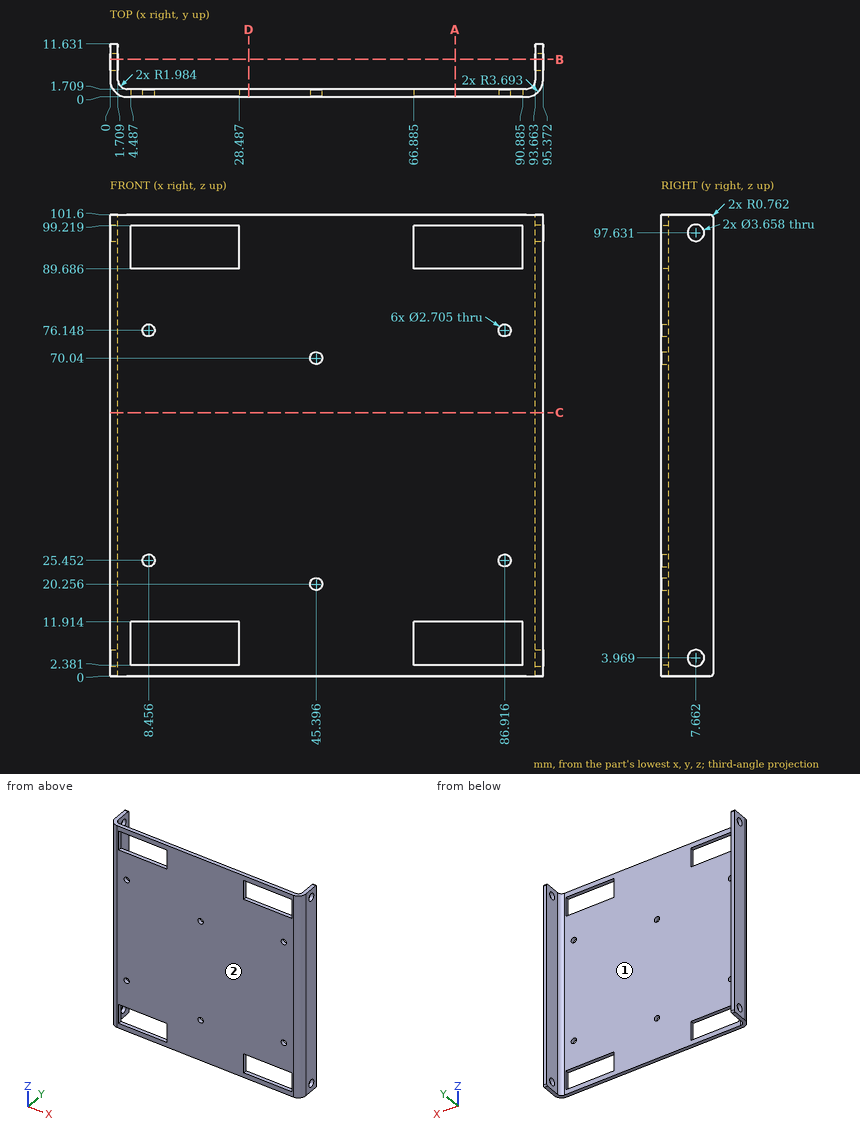
Verification items for this drawing (mm, ordinates from the low corner). Coordinates: 2 decimals unless noted, no trailing zeros. Write each loop counter-clockwise with the first axis right and the second up, starting at its lowest first coordinate (ties: lowest second). Pieces come first, ordered by that corner, then holes. Notation, with made-up numbers: M 33.25,-19 L 87.25,-19 A31 ccw 87.25,5 Z; hole C 7,29 d6. An arc over 180 degrees is marked long. Answer as a JSON object with one key per item and string values. Group by question number.
(1) Cross-section at D-D, the plane x = 30.5. Record the cut outline in (y, z).
(2) Cross-section at C-C, the plane z = 58. Record the cut outline in (x, y), and give its area (3 significant figures).
(3) Release check for a two-part mould opening along X. For the marked faces 1 and 2 record: +X half, -X half, draft (parallel to the pull), parting line (faces both ways), or undercut.
(4) Gauge pin test, flat ends, axial feed: pin 1 (1.4 mm diameter, centred on y = 0.5, z = 5, fed in from +X) (1 decimal); pin 2 (1.4 mm diameter, centred on y = 1, z = 93.5, fed in from +X); pin 3 (1.4 mm diameter, centred on y = 0.5, z = 8, fed in from -X). Record the tip position at first contact, or that the pin passes through.
(5) Cross-section at A-A, the plane x = 76. Record the cut outline in (y, z) (1 decimal).
(6) Cross-section at B-B, the plane y = 8.25. Record the cut outline in (x, z).
(7) Material ranges on line 1 (X direction, y = 4.75, z = 21.5); line 2 (Y direction, x = 64, z = 5); line 3 (X direction, y = 1, z = 95) (1 decimal), recorded low to high.
Reply:
{
 "1": {"outline": "M 0,0 L 1.71,0 L 1.71,101.6 L 0,101.6 Z"},
 "2": {"outline": "M 0,3.69 A3.69 ccw 3.69,0 L 91.68,0 A3.69 ccw 95.37,3.69 L 95.37,11.63 L 93.66,11.63 L 93.66,3.69 A1.98 cw 91.68,1.71 L 3.69,1.71 A1.98 cw 1.71,3.69 L 1.71,11.63 L 0,11.63 Z", "area": "193 mm²"},
 "3": {"face 1": "undercut", "face 2": "draft"},
 "4": {"pin 1": "x = 94.4", "pin 2": "x = 94.79", "pin 3": "x = 0.97"},
 "5": {"outline": "M 0,0 L 1.7,0 L 1.7,2.4 L 0,2.4 Z; M 0,11.9 L 1.7,11.9 L 1.7,89.7 L 0,89.7 Z; M 0,99.2 L 1.7,99.2 L 1.7,101.6 L 0,101.6 Z"},
 "6": {"outline": "M 0,0 L 1.71,0 L 1.71,2.24 L 0,2.24 Z; M 0,5.7 L 1.71,5.7 L 1.71,95.9 L 0,95.9 Z; M 0,99.36 L 1.71,99.36 L 1.71,101.6 L 0,101.6 Z; M 93.66,0 L 95.37,0 L 95.37,2.24 L 93.66,2.24 Z; M 93.66,5.7 L 95.37,5.7 L 95.37,95.9 L 93.66,95.9 Z; M 93.66,99.36 L 95.37,99.36 L 95.37,101.6 L 93.66,101.6 Z"},
 "7": {"line 1": "0 to 1.71, 93.66 to 95.37", "line 2": "0 to 1.71", "line 3": "1.2 to 4.5, 28.5 to 66.9, 90.9 to 94.2"}
}
